```python
from build123d import *

# Parameters (mm, degrees)
BOSS_EXTRUDE1_DEPTH = 10
SKETCH5_W           = 190.665965361
SKETCH5_H           = 98.914857752
CUT_EXTRUDE2_DEPTH  = 131.512395512
SKETCH3_W           = 191.984120241
SKETCH3_H           = 92.475390347
CUT_EXTRUDE1_DEPTH  = 125.356356188


with BuildPart() as part:
    # Sketch2 → Boss-Extrude1 (new body)
    with BuildSketch(Plane(origin=(0, 0, 0), x_dir=(1, 0, 0), z_dir=(0, 1, 0))):
        with BuildLine():
            Line((-26, 24.3), (0, 24.3))
            add(Edge.make_bspline(
                [(0, 24.3), (20.683832289, 24.384713811), (29.8, 14.098961604), (29.8, 0)],
                knots=[0, 0, 0, 0, 1, 1, 1, 1], degree=3))
            add(Edge.make_bspline(
                [(29.8, 0), (29.8, -15.903385672), (12.793782652, -19.673675204), (0, -22.5)],
                knots=[0, 0, 0, 0, 1, 1, 1, 1], degree=3))
            add(Edge.make_bspline(
                [(-86.5, -27.9), (-58.742591927, -27.9), (0, -22.5)],
                knots=[0, 0, 0, 1, 1, 1], degree=2))
            add(Edge.make_bspline(
                [(-124.6, 11.6), (-126.645501882, -15.929564791), (-96.169164371, -28.458925346), (-86.5, -27.9)],
                knots=[0, 0, 0, 0, 1, 1, 1, 1], degree=3))
            add(Edge.make_bspline(
                [(-86.5, 37.2), (-111.583343569, 37.2), (-124.6, 21.145918181), (-124.6, 11.6)],
                knots=[0, 0, 0, 0, 1, 1, 1, 1], degree=3))
            add(Edge.make_bspline(
                [(-26, 24.3), (-46.37360759, 24.3), (-60.223367409, 37.2), (-86.5, 37.2)],
                knots=[0, 0, 0, 0, 1, 1, 1, 1], degree=3))
        make_face()
    extrude(amount=BOSS_EXTRUDE1_DEPTH)

    # Sketch5 → Cut-Extrude2 (cut, through all)
    with BuildSketch(Plane(origin=(0, 10, 0), x_dir=(1, 0, 0), z_dir=(0, 1, 0))):
        with Locations((-37.807166851, 5.712427693)):
            Rectangle(SKETCH5_W, SKETCH5_H)
        with BuildLine():
            Line((0, 19.3), (-26, 19.3))
            add(Edge.make_bspline(
                [(-26, 19.3), (-28.614389566, 19.3), (-31.195480065, 19.494126305), (-36.299918034, 20.219008193), (-38.823236595, 20.749932309), (-43.82844627, 22.053293526), (-46.31311575, 22.826190042), (-51.244397222, 24.470393512), (-53.69402913, 25.341112046), (-58.607069123, 27.040712597), (-61.070722849, 27.868848632), (-64.806301572, 28.989279687), (-66.059451522, 29.343006622), (-68.572193461, 29.996166113), (-69.832412317, 30.295833479), (-73.626302931, 31.102275727), (-76.173387066, 31.51524352), (-81.307214737, 32.063798503), (-83.893870441, 32.2), (-86.5, 32.2)],
                knots=[0, 0, 0, 0, 0.125, 0.125, 0.25, 0.25, 0.375, 0.375, 0.5, 0.5, 0.625, 0.625, 0.6875, 0.6875, 0.75, 0.75, 0.875, 0.875, 1, 1, 1, 1], degree=3))
            add(Edge.make_bspline(
                [(-86.5, 32.2), (-90.047671723, 32.2), (-93.539315109, 31.853363621), (-97.818101716, 30.88944061), (-98.669522164, 30.669824618), (-100.363040922, 30.17291839), (-101.207876089, 29.89460231), (-103.707194596, 28.9730152), (-105.314538731, 28.24898707), (-108.402461221, 26.564840966), (-109.885156962, 25.604040465), (-112.695415045, 23.412360835), (-113.989352092, 22.209304545), (-115.736354807, 20.217749989), (-116.286105675, 19.522480074), (-117.307591473, 18.056713662), (-117.771937921, 17.297113036), (-118.380597746, 16.112260348), (-118.568848857, 15.709499136), (-118.910400222, 14.885324985), (-119.063856456, 14.46298862), (-119.32099023, 13.612441675), (-119.425833719, 13.182501201), (-119.534502641, 12.528030347), (-119.56255262, 12.308265558), (-119.588853411, 11.975515189), (-119.594973106, 11.86407762), (-119.600932982, 11.639967141), (-119.6, 11.527142129), (-119.6, 11.414500659)],
                knots=[0, 0, 0, 0, 0.25, 0.25, 0.3125, 0.3125, 0.375, 0.375, 0.5, 0.5, 0.625, 0.625, 0.75, 0.75, 0.8125, 0.8125, 0.875, 0.875, 0.90625, 0.90625, 0.9375, 0.9375, 0.96875, 0.96875, 0.984375, 0.984375, 0.9921875, 0.9921875, 1, 1, 1, 1], degree=3))
            add(Edge.make_bspline(
                [(-119.6, 11.414500659), (-119.620469876, 11.139005048), (-119.640012507, 10.863585734), (-119.66949801, 10.313536999), (-119.702590259, 9.489380197), (-119.701746238, 8.668015761), (-119.653311171, 7.029133356), (-119.558725583, 5.941670929), (-119.316814989, 4.318708201), (-119.219497862, 3.779093122), (-118.990298597, 2.702707063), (-118.857842254, 2.164001324), (-118.411370332, 0.568296748), (-118.049576648, -0.466050211), (-117.204822005, -2.479103419), (-116.721870667, -3.457814087), (-115.911016092, -4.886192051), (-115.626316263, -5.355698602), (-115.028686616, -6.281748331), (-114.715117794, -6.739029825), (-113.098128241, -8.967198862), (-111.636582687, -10.586754888), (-109.243370012, -12.821144966), (-108.411754958, -13.533067597), (-107.116844881, -14.554870601), (-106.676456633, -14.888333255), (-105.787025552, -15.535321816), (-105.337421344, -15.84934205), (-103.066112758, -17.374312871), (-101.175798147, -18.452299517), (-98.237583629, -19.870168351), (-97.240844592, -20.309198302), (-95.209999189, -21.114841784), (-94.174615133, -21.48224539), (-92.064314636, -22.126795927), (-91.001033475, -22.402007075), (-89.387886633, -22.70933152), (-88.84713932, -22.794224632), (-88.028751145, -22.879499568), (-87.754740398, -22.90089357), (-87.340882626, -22.916536257), (-87.202453029, -22.918989427), (-86.924204685, -22.915854968), (-86.784006393, -22.908070411), (-86.64375233, -22.899963035)],
                knots=[0, 0, 0, 0, 0.015625, 0.015625, 0.03125, 0.0625, 0.0625, 0.125, 0.125, 0.15625, 0.15625, 0.1875, 0.1875, 0.25, 0.25, 0.3125, 0.3125, 0.34375, 0.34375, 0.375, 0.375, 0.5, 0.5, 0.5625, 0.5625, 0.59375, 0.59375, 0.625, 0.625, 0.75, 0.75, 0.8125, 0.8125, 0.875, 0.875, 0.9375, 0.9375, 0.96875, 0.96875, 0.984375, 0.984375, 0.9921875, 0.9921875, 1, 1, 1, 1], degree=3))
            add(Edge.make_bspline(
                [(-86.64375233, -22.899963035), (-83.051721737, -22.901813131), (-79.463866007, -22.836654879), (-72.292852573, -22.630933055), (-68.709770334, -22.489158228), (-57.965349536, -21.986375675), (-50.808741052, -21.549448214), (-36.50252062, -20.563295893), (-29.353030187, -20.012120654), (-15.058799553, -18.833526914), (-7.914092044, -18.205583695), (-0.771119947, -17.549786375)],
                knots=[0, 0, 0, 0, 0.125, 0.125, 0.25, 0.25, 0.5, 0.5, 0.75, 0.75, 1, 1, 1, 1], degree=3))
            add(Edge.make_bspline(
                [(-0.771119947, -17.549786375), (1.963321139, -16.94544861), (4.695341149, -16.33357579), (8.730024902, -15.218615637), (10.064478195, -14.814466089), (12.699729823, -13.90142355), (14.000796007, -13.393364173), (15.911888282, -12.505206219), (16.542091865, -12.187905528), (17.784402153, -11.496981701), (18.391917697, -11.125662576), (19.559410174, -10.32463286), (20.121164342, -9.894098151), (20.920538613, -9.18924898), (21.180682911, -8.943393186), (21.678462153, -8.434660622), (21.916135354, -8.171907904), (22.59259098, -7.356311131), (22.994745994, -6.776081028), (23.513123046, -5.842290056), (23.671822244, -5.519779327), (23.953566298, -4.86813842), (24.077688222, -4.537273262), (24.402854637, -3.53046254), (24.556745878, -2.840315617), (24.755950633, -1.42732092), (24.8, -0.714331591), (24.8, 0)],
                knots=[0, 0, 0, 0, 0.25, 0.25, 0.375, 0.375, 0.5, 0.5, 0.5625, 0.5625, 0.625, 0.625, 0.6875, 0.6875, 0.71875, 0.71875, 0.75, 0.75, 0.8125, 0.8125, 0.84375, 0.84375, 0.875, 0.875, 0.9375, 0.9375, 1, 1, 1, 1], degree=3))
            add(Edge.make_bspline(
                [(24.8, 0), (24.800001574, 1.499794527), (24.679867583, 2.978315628), (24.270262238, 5.1554747), (24.095205029, 5.874372955), (23.764785291, 6.940708409), (23.64330548, 7.294145508), (23.375491288, 7.996618496), (23.229208001, 8.345127218), (22.758435322, 9.365838107), (22.399931747, 10.019031745), (21.589242675, 11.268187742), (21.136243882, 11.865038785), (19.63468306, 13.559968632), (18.489202915, 14.513686307), (16.909680401, 15.525653475), (16.58535259, 15.719500417), (15.929822317, 16.085938782), (15.598164332, 16.258912353), (14.592578593, 16.74990385), (13.908081512, 17.040104299), (12.515293354, 17.557881638), (11.806985872, 17.785415353), (10.369782811, 18.186296846), (9.638661479, 18.360025682), (7.436633609, 18.806009812), (5.959001697, 19.004489088), (2.98950105, 19.255065786), (1.497532001, 19.3061318), (0, 19.3)],
                knots=[0, 0, 0, 0, 0.125, 0.125, 0.1875, 0.1875, 0.21875, 0.21875, 0.25, 0.25, 0.3125, 0.3125, 0.375, 0.375, 0.5, 0.5, 0.53125, 0.53125, 0.5625, 0.5625, 0.625, 0.625, 0.6875, 0.6875, 0.75, 0.75, 0.875, 0.875, 1, 1, 1, 1], degree=3))
        make_face(mode=Mode.SUBTRACT)
    extrude(amount=-CUT_EXTRUDE2_DEPTH, mode=Mode.SUBTRACT)

    # Sketch3 → Cut-Extrude1 (cut, through all)
    with BuildSketch(Plane(origin=(0, 10, 0), x_dir=(1, 0, 0), z_dir=(0, 1, 0))):
        with Locations((-40.989040218, 1.022012658)):
            Rectangle(SKETCH3_W, SKETCH3_H)
        with BuildLine():
            Line((0, 19.3), (0, 10.258653745))
            ThreePointArc((0, 10.258653745), (10.258653745, 0), (0, -10.258653745))
            Line((0, -10.258653745), (-0.771119947, -17.549786375))
            add(Edge.make_bspline(
                [(-0.771119947, -17.549786375), (1.963321139, -16.94544861), (4.695341149, -16.33357579), (8.730024902, -15.218615637), (10.064478195, -14.814466089), (12.699729823, -13.90142355), (14.000796007, -13.393364173), (15.911888282, -12.505206219), (16.542091865, -12.187905528), (17.784402153, -11.496981701), (18.391917697, -11.125662576), (19.559410174, -10.32463286), (20.121164342, -9.894098151), (20.920538613, -9.18924898), (21.180682911, -8.943393186), (21.678462153, -8.434660622), (21.916135354, -8.171907904), (22.59259098, -7.356311131), (22.994745994, -6.776081028), (23.513123046, -5.842290056), (23.671822244, -5.519779327), (23.953566298, -4.86813842), (24.077688222, -4.537273262), (24.402854637, -3.53046254), (24.556745878, -2.840315617), (24.755950633, -1.42732092), (24.8, -0.714331591), (24.8, 0)],
                knots=[0, 0, 0, 0, 0.25, 0.25, 0.375, 0.375, 0.5, 0.5, 0.5625, 0.5625, 0.625, 0.625, 0.6875, 0.6875, 0.71875, 0.71875, 0.75, 0.75, 0.8125, 0.8125, 0.84375, 0.84375, 0.875, 0.875, 0.9375, 0.9375, 1, 1, 1, 1], degree=3))
            add(Edge.make_bspline(
                [(24.8, 0), (24.800001574, 1.499794527), (24.679867583, 2.978315628), (24.270262238, 5.1554747), (24.095205029, 5.874372955), (23.764785291, 6.940708409), (23.64330548, 7.294145508), (23.375491288, 7.996618496), (23.229208001, 8.345127218), (22.758435322, 9.365838107), (22.399931747, 10.019031745), (21.589242675, 11.268187742), (21.136243882, 11.865038785), (19.63468306, 13.559968632), (18.489202915, 14.513686307), (16.909680401, 15.525653475), (16.58535259, 15.719500417), (15.929822317, 16.085938782), (15.598164332, 16.258912353), (14.592578593, 16.74990385), (13.908081512, 17.040104299), (12.515293354, 17.557881638), (11.806985872, 17.785415353), (10.369782811, 18.186296846), (9.638661479, 18.360025682), (7.436633609, 18.806009812), (5.959001697, 19.004489088), (2.98950105, 19.255065786), (1.497532001, 19.3061318), (0, 19.3)],
                knots=[0, 0, 0, 0, 0.125, 0.125, 0.1875, 0.1875, 0.21875, 0.21875, 0.25, 0.25, 0.3125, 0.3125, 0.375, 0.375, 0.5, 0.5, 0.53125, 0.53125, 0.5625, 0.5625, 0.625, 0.625, 0.6875, 0.6875, 0.75, 0.75, 0.875, 0.875, 1, 1, 1, 1], degree=3))
        make_face(mode=Mode.SUBTRACT)
    extrude(amount=-CUT_EXTRUDE1_DEPTH, mode=Mode.SUBTRACT)


solid = part.part
```
Could you check a few things on this model? Use its own coordinates, in mm. A direction names the side the tool comes from. Round coordinates to 2 decimals unless told otherwise and drop trailing zeros. Answer in a Markdown table with one row per item. Add a question column.
Q1. On a 3-axis mill with a long thin cutter (end or side, diameter ignored), from which of +Z, -Z, +X, -X, +Y, -Y can I reach the whole of each face in a straight line? I mean faces 4 (the flat face through (0, 5, -15)), 5 (the flat face through (12, 0, -1)). Say none if no direction works.
Q2. If we mould it in two halves opening along Z, with no side actions, what happens to faces 1 (the cylindrical face through (10.256, 5.07, -0.226)), 2 (the flat face through (12, 10, -1)), 3 (the flat face through (-0.38, 5.07, 13.85))? For each: +Z half, -Z half, draft (parallel to the pull), parting line (faces both ways), or undercut.
Q3. Will these pins go through, and if not, where does the flat tip stop? pin 1 Ø4.5 at (y, z) = (4, -14.5) entering from -X; pin 2 Ø2 at (x, y) = (5, 4.5) entering from -Z; pin 3 Ø4 at (y, z) = (5.5, -15) entering from +X.
Q4. If I drill on line 1 (Z direction, x = 1.5, y = 5); line 2 (Z direction, x = 7.75, y = 1); line 3 (X direction, y = 5.25, z = -16.5), over which ranges is the centre line in solid material (lowest first)? Write a range as from..to.
Values:
| question | item | result |
|---|---|---|
| 1 | face 4 | -Z, -X, +Y, -Y |
| 1 | face 5 | +Z, -Z, +X, -X, -Y |
| 2 | face 1 | undercut |
| 2 | face 2 | draft |
| 2 | face 3 | -Z half |
| 3 | pin 1 | x = 0 |
| 3 | pin 2 | z = -19.17 |
| 3 | pin 3 | x = 20.1 |
| 4 | line 1 | -19.29..-10.15, 10.15..17.04 |
| 4 | line 2 | -18.72..-6.72, 6.72..15.49 |
| 4 | line 3 | 0..15.1 |
